```python
from build123d import *

# Parameters (mm, degrees)
BOX049_W     = 10
BOX049_H     = 10
BOX049_DEPTH = 130
BOX050_W     = 10
BOX050_H     = 115
BOX050_DEPTH = 10
BOX051_W     = 10
BOX051_H     = 115
BOX051_DEPTH = 10
BOX048_W     = 10
BOX048_H     = 10
BOX048_DEPTH = 130


with BuildPart() as cubo012:
    # Box049 → Box049 (new body)
    with BuildSketch(Plane(origin=(-37, 115, 15), x_dir=(1, 0, 0), z_dir=(0, 0, 1))):
        with Locations((5, 5)):
            Rectangle(BOX049_W, BOX049_H)
    extrude(amount=BOX049_DEPTH)


with BuildPart() as cubo013:
    # Box050 → Box050 (new body)
    with BuildSketch(Plane(origin=(-37, 115, 145), x_dir=(1, 0, 0), z_dir=(0, 0, 1))):
        with Locations((5, 57.5)):
            Rectangle(BOX050_W, BOX050_H)
    extrude(amount=BOX050_DEPTH)


with BuildPart() as cubo014:
    # Box051 → Box051 (new body)
    with BuildSketch(Plane(origin=(-37, 115, 5), x_dir=(1, 0, 0), z_dir=(0, 0, 1))):
        with Locations((5, 57.5)):
            Rectangle(BOX051_W, BOX051_H)
    extrude(amount=BOX051_DEPTH)


with BuildPart() as fusion007:
    # Box048 → Box048 (new body)
    with BuildSketch(Plane(origin=(-37, 220, 15), x_dir=(1, 0, 0), z_dir=(0, 0, 1))):
        with Locations((5, 5)):
            Rectangle(BOX048_W, BOX048_H)
    extrude(amount=BOX048_DEPTH)

    # Fusion007: union Cubo012, Cubo013, Cubo014
    add(cubo012.part)
    add(cubo013.part)
    add(cubo014.part)


with BuildPart() as fusion007_1:
    # Fusion007 placement: moved
    add(fusion007.part.moved(Location((26.5, -253, 1))))


solid = fusion007_1.part
```
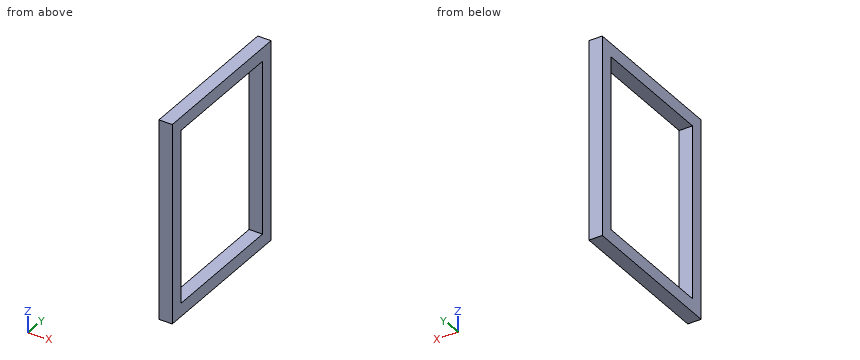
Source: CAD feature listing. Evaluate the final solid. Frame: model axes, mm. Coordinates: 2 decimals unless noted, no trailing zeros. Loops run counter-clockwise (first coordinate to the right, second up) from the corner with the lowest first, then second, coordinate; pieces in that order, holes last. Notation, with made-up numbers: M -34,6.5 L 14,6.5 A30 ccw 14,31.5 Z; hole C 64,-10 d9. An arc over 180 degrees is marked long. Use CSV: the item, a comma, the result in double quotes.
(1) Cut plane A-A on z = 112. Return loops of the section in (x, y), and give its area (3 significant figures).
Answers follow:
outline,"M -10.5,-138 L -0.5,-138 L -0.5,-128 L -10.5,-128 Z; M -10.5,-33 L -0.5,-33 L -0.5,-23 L -10.5,-23 Z"
area,"200 mm²"
(2) Line query: line 1 (Y direction, x = -4, z = 30); line 2 (Z direction, x = -5, y = -64). Output: solid intervals per line, ascending. Write a range as [from, to].
Answers follow:
line 1,"[-138, -128], [-33, -23]"
line 2,"[6, 16], [146, 156]"
(3) Cut plane B-B on y = -48. Return loops of the section in (x, z).
Answers follow:
outline,"M -10.5,6 L -0.5,6 L -0.5,16 L -10.5,16 Z; M -10.5,146 L -0.5,146 L -0.5,156 L -10.5,156 Z"
(4) Cut plane C-C on x = -5.25. Return loops of the section in (y, z), and give its area (3 significant figures).
Answers follow:
outline,"M -138,6 L -23,6 L -23,156 L -138,156 Z; hole M -128,16 L -33,16 L -33,146 L -128,146 Z"
area,"4,900 mm²"
